Geometry check sheet. Reference: the model listing, model coordinates, mm. Coordinates: 2 decimals unless noted, no trailing zeros. Write each loop counter-clockwise with the first axis right and the second up, starting at its lowest first coordinate (ties: lowest second). Pieces come first, ordered by that corner, then holes. Notation, with made-up numbers: (-36, 50.25) -> (-19, 50.25) arc R19 cw to (-19, 72.25) -> close; hole circle Ø10 at (85, 89.25). An arc over 180 degrees is marked (long way). One line per question, with ' | ' between items.
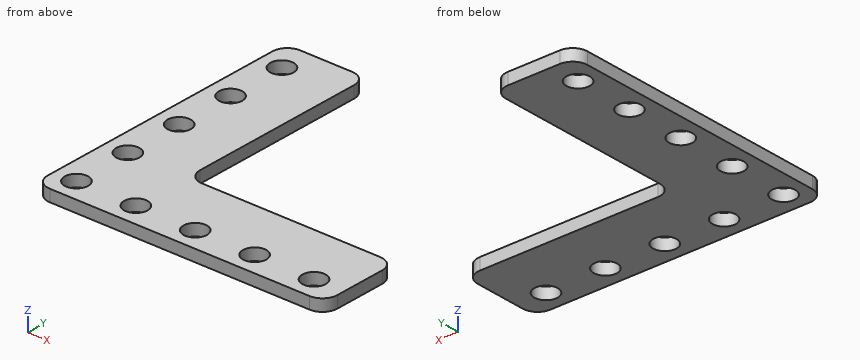
Autodesk Inventor part; units mm, degrees
ref_plane "YZ Plane" through (0, 0, 0) normal (1, 0, 0) x (0, 1, 0)
ref_plane "XZ Plane" through (0, 0, 0) normal (0, 1, 0) x (-1, 0, 0)
ref_plane "XY Plane" through (0, 0, 0) normal (0, 0, 1) x (1, 0, 0)
sketch "Sketch1" plane through (0, 0, 0) normal (0, 0, 1) x (1, 0, 0)
  line L0 (0, 0) -> (0, 69.85) construction
  line L1 (0, 69.85) -> (7.9375, 69.85) construction
  line L2 (7.9375, 69.85) -> (7.9375, 0) construction
  line L3 (7.9375, 69.85) -> (25.4, 69.85)
  line L4 (25.4, 69.85) -> (25.4, 17.4625)
  line L5 (25.4, 17.4625) -> (69.85, 17.4625)
  line L6 (69.85, 0) -> (0, 0) construction
  line L7 (25.4, 25.4) -> (69.85, 25.4)
  line L8 (69.85, 25.4) -> (69.85, 17.4625)
  circle A0 centre (12.7, 63.5) radius 2.4892
  circle A1 centre (12.7, 50.8) radius 2.4892
  circle A2 centre (12.7, 38.1) radius 2.4892
  circle A3 centre (12.7, 25.4) radius 2.4892
  circle A4 centre (12.7, 12.7) radius 2.4892
  circle A5 centre (25.4, 12.7) radius 2.4892
  circle A6 centre (38.1, 12.7) radius 2.4892
  circle A7 centre (50.8, 12.7) radius 2.4892
  circle A8 centre (63.5, 12.7) radius 2.4892
  line L9 (69.85, 7.9375) -> (7.9375, 7.9375)
  line L10 (69.85, 17.4625) -> (69.85, 7.9375)
  line L11 (69.85, 7.9375) -> (69.85, 0) construction
  line L12 (7.9375, 69.85) -> (7.9375, 7.9375)
  line L13 (12.7, 63.5) -> (12.7, 50.8) construction
  point P0 (16.6687, 69.85)
  dimension "d0" = 17.4625
  dimension "d3" = 25.4
  dimension "d4" = 4.9784
  dimension "d7" = 12.7
  dimension "d12" = 6.35
  dimension "d15" = 12.7
  dimension "d22" = 12.7
  dimension "d23" = 9.525
  dimension "d24" = 6.35
  dimension "d30" = 25.4
  dimension "d31" = 4.7625
extrude "Extrusion1" add sketch "Sketch1" along normal mid plane 2.5 contours L3 L4 L5 L10 L9 L12
extrude "Extrusion2" add sketch "Sketch1" along normal mid plane 2.5 contours L7 L8 L5 L4
fillet "Fillet1" radius 3.175 6 edges at (25.4, 69.85, 0) (7.9375, 69.85, 0) (7.9375, 7.9375, 0) (69.85, 7.9375, 0) (69.85, 25.4, 0) (25.4, 25.4, 0)
properties part number "TTB Elevator L Gussets"
(1) Cross-section at B-B (y = 12.7). Record the cut outline in (x, z), plus the area to 3 significant figures.
Answers below:
outline: (7.94, -1.25) -> (10.21, -1.25) -> (10.21, 1.25) -> (7.94, 1.25) -> close; (15.19, -1.25) -> (22.91, -1.25) -> (22.91, 1.25) -> (15.19, 1.25) -> close; (27.89, -1.25) -> (35.61, -1.25) -> (35.61, 1.25) -> (27.89, 1.25) -> close; (40.59, -1.25) -> (48.31, -1.25) -> (48.31, 1.25) -> (40.59, 1.25) -> close; (53.29, -1.25) -> (61.01, -1.25) -> (61.01, 1.25) -> (53.29, 1.25) -> close; (65.99, -1.25) -> (69.85, -1.25) -> (69.85, 1.25) -> (65.99, 1.25) -> close | area: 92.6 mm²
(2) Material ranges on line 1 (Y direction, x = 12.7, z = 0.05); line 2 (X direction, y = 11.5, z = 1); line 3 (Y direction, x = 63.5, z = 0.1), recorded low to high.
Answers below:
line 1: y = 7.94 to 10.21, 15.19 to 22.91, 27.89 to 35.61, 40.59 to 48.31, 53.29 to 61.01, 65.99 to 69.85 | line 2: x = 7.94 to 10.52, 14.88 to 23.22, 27.58 to 35.92, 40.28 to 48.62, 52.98 to 61.32, 65.68 to 69.85 | line 3: y = 7.94 to 10.21, 15.19 to 25.4
(3) Depth check by flat-ended pin: P1, Ø4.5, axis at x = 25.4, y = 12.7, coming from the +Z side; P2, Ø0.8, axis at x = 48, z = 0, coming from the +Y side; P3, Ø6.5, axis at x = 50.8, y = 12.7, coming from the -Z side; P4, Ø1, axis at y = 55.5, z = -0.5, coming from the +X side. Enter the tip coordinate at first touch or a pass-through.
Answers below:
P1: passes through | P2: stops at y = 25.4 | P3: stops at z = -1.25 | P4: stops at x = 25.4
(4) Cross-section at A-A (x = 63.5). Record the cut outline in (y, z).
Answers below:
outline: (7.94, -1.25) -> (10.21, -1.25) -> (10.21, 1.25) -> (7.94, 1.25) -> close; (15.19, -1.25) -> (25.4, -1.25) -> (25.4, 1.25) -> (15.19, 1.25) -> close
(5) Cross-section at D-D (z = 0.15). Count the separate pieces of the cut face and the enclosed holes in it, plus the area to 3 significant figures.
Answers below:
separate pieces: 1 | enclosed holes: 9 | area: 1,670 mm²
